For this review, take the finished solid that the model builds, in its own axes (mm). A direction names the side the tool comes from. Round coordinates to 2 decimals unless told otherwise and drop trailing zeros. Loops run counter-clockwise (first coordinate to the right, second up) from the corner with the lowest first, then second, coordinate; pieces in that order, holes last.
1. Consider section A-A on x = 0. State the section outline as (y, z) points.
2. Clearance check with flat-ended pins moving along their axes: pin 1 Ø3 at (x, y) = (-4.5, 4.5) entering from -Z; pin 2 Ø3 at (x, y) = (12.5, 3.5) entering from +Z; pin 3 Ø3 at (x, y) = (5, 13) entering from +Z. State where each tip first meets the part, or that it passes through.
3. Consider section C-C on y = -4.5. State the section outline as (x, z) points, then the cut area to 3 significant figures.
4. Draft analysis for pull direction Z (two halves, no side actions). For faces 1 (the flat face through (-22, 0, 14)), 2 (the cylindrical face through (0.9, 36.91, 2.86)), state which applies: released by +Z, released by -Z, zero draft, split by the parting line, or undercut.
5. To check wall thickness, follow line 1 along Y through (x, z) = (-7, 25.5); line 2 along Y through (x, z) = (10.5, 11); line 3 along X through (y, z) = (22, 3.5). State the ranges of each line that lie inside material, in increasing order.
6. Tool access review of faces 3 (the cylindrical face through (9.76, -4.93, 31)), 4 (the flat face through (1, 27.05, 3)): name each direction out of +Z, -Z, +X, -X, +Y, -Y from which nothing blocks a thin tool from reaching the whole face with its end or side.
7. Consider section B-B on y = 36.5. State the section outline as (x, z) points.
from build123d import *

# Parameters (mm, degrees)
SKETCH_2_R      = 6.56
SKETCH_1_R      = 25.5
SKETCH_3_R      = 32.5
EXTRUDE_1_DEPTH = 10
SKETCH_4_R      = 3
EXTRUDE_2_DEPTH = 20


with BuildPart() as part:
    # 스케치2 → 로프트1 section 0
    with BuildSketch(Plane(origin=(0, 27.05, 0), x_dir=(1, 0, 0), z_dir=(0, 1, 0))):
        Circle(SKETCH_2_R)
    # 스케치1 → 로프트1 section 1
    with BuildSketch(Plane(origin=(0, 0, 0), x_dir=(1, 0, 0), z_dir=(0, 1, 0))):
        Circle(SKETCH_1_R)
    loft()

    # 스케치3 → 보스-돌출1 (add)
    with BuildSketch(Plane(origin=(0, 0, 0), x_dir=(1, 0, 0), z_dir=(0, 1, 0))):
        with Locations(Location((0, 0, 0), (0, 0, 270))):
            Circle(SKETCH_3_R)
    extrude(amount=-EXTRUDE_1_DEPTH)

    # 스케치4 → 보스-돌출2 (add)
    with BuildSketch(Plane(origin=(0, 27.05, 0), x_dir=(1, 0, 0), z_dir=(0, 1, 0))):
        with Locations(Location((0, 0, 0), (0, 0, 270))):
            Circle(SKETCH_4_R)
    extrude(amount=EXTRUDE_2_DEPTH)


solid = part.part
Resolved:
1. outline: (-10, -32.5) - (0, -32.5) - (0, -25.5) - (27.05, -6.56) - (27.05, -3) - (47.05, -3) - (47.05, 3) - (27.05, 3) - (27.05, 6.56) - (0, 25.5) - (0, 32.5) - (-10, 32.5) - close
2. pin 1: stops at z = -23
2. pin 2: stops at z = 20.89
2. pin 3: stops at z = 16.8
3. outline: circle Ø65 at (0, 0)
3. area: 3,320 mm2
4. face 1: zero draft
4. face 2: split by the parting line
5. line 1: y = -10 to 0
5. line 2: y = -10 to 14.7
5. line 3: x = -9.47 to 9.47
6. face 3: +Y, -Y
6. face 4: +Y
7. outline: circle Ø6 at (0, 0)
